from build123d import *

# Parameters (mm, degrees)
EXTRUDE_1_DEPTH = 15
EXTRUDE_START   = 8
EXTRUDE_3_DEPTH = 7
EXTRUDE_4_DEPTH = 15
EXTRUDE_5_DEPTH = 15
EXTRUDE_6_DEPTH = 15
FILLET_1_R      = 2
FILLET_2_R      = 0.8
F_2_0MM_1_D     = 2.2
F_2_0MM_1_DEPTH = 1.5
F_2_0MM_1_TIP   = 0.660946681
F_2_0MM_2_D     = 2.2
F_2_0MM_2_DEPTH = 1.5
F_2_0MM_2_TIP   = 0.660946681


with BuildPart() as part:
    # 草图1 → 凸台-拉伸1 (new body)
    with BuildSketch(Plane(origin=(0, 0, 0), x_dir=(1, 0, 0), z_dir=(0, 1, 0))):
        Polygon((49.5194763, 27.3201645), (0, 0), (14.2759212, -89.0995664), (44.3217232, -113.2519378), (135.6782768, -113.2519378), (165.7240788, -89.0995664), (180, 0), (130.4805237, 27.3201645), (90, 17.2995935), align=None)
        Polygon((6.502592683, -14.920940874), (11.7659704, -11.9027565), (24.4692995, -92.1170773), (17.9120995, -86.965507524), align=None, mode=Mode.SUBTRACT)
        Polygon((51.5112815, 10), (90, 0), (128.4887185, 10), (152.140164487, -3.156709279), (153.941562556, -4.158782079), (157.3669305, -6.0642288), (164.466088374, -10.013313195), (163.0222846, -19.1574054), (162.41503493, -23.003320662), (162.112651759, -24.918414423), (150.9253582, -95.7712863), (134.2722611, -109.1590702), (45.7277389, -109.1590702), (29.0746418, -95.7712863), (17.887348241, -24.918414423), (17.58496507, -23.003320662), (16.9777154, -19.1574054), (15.533911626, -10.013313195), (22.6330695, -6.0642288), (26.058437444, -4.158782079), (27.859835513, -3.156709279), align=None, mode=Mode.SUBTRACT)
        Polygon((162.0879005, -86.965507524), (155.5307005, -92.1170773), (168.2340296, -11.9027565), (173.497407317, -14.920940874), align=None, mode=Mode.SUBTRACT)
        Polygon((50.326908, 23.3565545), (90, 13.1373278), (129.673092, 23.3565545), (166.5422291, 2.924677806), (165.312614852, -5.602660324), (128.635248263, 14.72294235), (90, 4.7710495), (51.364751737, 14.72294235), (14.687385148, -5.602660324), (13.4577709, 2.924677806), align=None, mode=Mode.SUBTRACT)
    extrude(amount=EXTRUDE_1_DEPTH)

    # 草图1<4> → 凸台-拉伸3 (add)
    with BuildSketch(Plane(origin=(0, 0, 0), x_dir=(1, 0, 0), z_dir=(0, 1, 0)).offset(EXTRUDE_START)):
        Polygon((164.466088374, -10.013313195), (163.0222846, -19.1574054), (155.8678549, -15.177574667), (157.3669305, -6.0642288), align=None)
        Polygon((153.941562556, -4.158782079), (152.140164487, -3.156709279), (149.6966334, -18.0116932), (162.112651759, -24.918414423), (162.41503493, -23.003320662), (151.8119905, -17.1051116), align=None)
        Polygon((22.6330695, -6.0642288), (15.533911626, -10.013313195), (16.9777154, -19.1574054), (24.1321451, -15.177574667), align=None)
        Polygon((30.3033666, -18.0116932), (27.859835513, -3.156709279), (26.058437444, -4.158782079), (28.1880095, -17.1051116), (17.58496507, -23.003320662), (17.887348241, -24.918414423), align=None)
    extrude(amount=EXTRUDE_3_DEPTH)

    # 草图3 → 凸台-拉伸4 (add)
    with BuildSketch(Plane(origin=(0, 0, 0), x_dir=(1, 0, 0), z_dir=(0, 1, 0))):
        Polygon((115.878940082, 32.456095876), (121.872227157, 33.965105872), (122.289100924, 40.131370332), (125.576282273, 34.897725339), (131.569569347, 36.406735336), (127.607872073, 31.663154849), (130.895053422, 26.429509857), (125.159408505, 28.73146088), (121.197711231, 23.987880393), (121.614584999, 30.154144853), align=None)
    extrude(amount=EXTRUDE_4_DEPTH)

    # 草图4 → 凸台-拉伸5 (add)
    with BuildSketch(Plane(origin=(0, 0, 0), x_dir=(1, 0, 0), z_dir=(0, 1, 0))):
        Polygon((168.625201424, 5.109151957), (158.192316311, 27.022904619), (179.513278304, 15.426602313), (155.448122239, 12.276060926), (173.065400703, 28.970046279), align=None)
        Polygon((173.065400703, 28.970046279), (166.336199119, 22.593511282), (171.369395495, 19.85599565), align=None)
        Polygon((179.513278304, 15.426602313), (171.369395495, 19.85599565), (170.321206632, 14.223202586), align=None)
        Polygon((170.321206632, 14.223202586), (164.640193911, 13.479460653), (168.625201424, 5.109151957), align=None)
        Polygon((164.640193911, 13.479460653), (162.177323823, 18.652595923), (155.448122239, 12.276060926), align=None)
        Polygon((166.336199119, 22.593511282), (158.192316311, 27.022904619), (162.177323823, 18.652595923), align=None)
    extrude(amount=EXTRUDE_5_DEPTH)

    # 草图5 → 凸台-拉伸6 (add)
    with BuildSketch(Plane(origin=(0, 0, 0), x_dir=(1, 0, 0), z_dir=(0, 1, 0))):
        Polygon((145.437967888, 18.068925838), (136.74389696, 36.330386388), (154.511365288, 26.666801134), (134.457068567, 24.041349978), (149.138133954, 37.953004439), align=None)
        Polygon((143.530465967, 32.639225275), (136.74389696, 36.330386388), (140.064736554, 29.355129142), align=None)
        Polygon((149.138133954, 37.953004439), (143.530465967, 32.639225275), (147.724796281, 30.357962248), align=None)
        Polygon((154.511365288, 26.666801134), (147.724796281, 30.357962248), (146.851305561, 25.663968028), align=None)
        Polygon((146.851305561, 25.663968028), (142.117128294, 25.044183084), (145.437967888, 18.068925838), align=None)
        Polygon((142.117128294, 25.044183084), (140.064736554, 29.355129142), (134.457068567, 24.041349978), align=None)
    extrude(amount=EXTRUDE_6_DEPTH)

    # 圆角1
    # the kernel refuses this fillet: 2 mm, written as the material it adds along each edge
    with BuildSketch(Plane(origin=(121.268833448, 15, -25.039897652), x_dir=(-0.9707016379334082, 0, 0.2402880149183444), z_dir=(0, -1, 0))) as fillet_1_piece_1:
        with BuildLine():
            CenterArc((FILLET_1_R * 0.72959801192, FILLET_1_R), FILLET_1_R, 197.771167986, 72.228832014)
            Line((-FILLET_1_R * 0.222685090293, FILLET_1_R * 0.69478385816), (-FILLET_1_R * 0.241730752337, FILLET_1_R * 0.688679535323))
            Line((-FILLET_1_R * 0.241730752337, FILLET_1_R * 0.688679535323), (-FILLET_1_R * 0.0145919602384, -FILLET_1_R * 0.02))
            Line((-FILLET_1_R * 0.0145919602384, -FILLET_1_R * 0.02), (FILLET_1_R * 0.72959801192, -FILLET_1_R * 0.02))
            Line((FILLET_1_R * 0.72959801192, -FILLET_1_R * 0.02), (FILLET_1_R * 0.72959801192, 0))
        make_face()
    extrude(amount=15)
    with BuildSketch(Plane(origin=(130.355139653, 0, -27.289126864), x_dir=(-0.5318771148973955, 0, -0.8468215482900885), z_dir=(0, 1, 0))) as fillet_1_piece_2:
        with BuildLine():
            CenterArc((0.649299153, -2), FILLET_1_R, 90, 20.172783533)
            Line((-0.040405567, -0.122686121), (-0.054199661, -0.085139844))
            ThreePointArc((-0.054199661, -0.085139844), (-0.058195374, -0.048830544), (-0.03799259, 0.012512517))
            Line((-0.03799259, 0.012512517), (0, 0.04))
            Line((0, 0.04), (0.649299153, 0.04))
            Line((0.649299153, 0.04), (0.649299153, 0))
        make_face()
    extrude(amount=15)
    with BuildSketch(Plane(origin=(168.822041947, 0, -6.166940275), x_dir=(0.18294627145075168, 0, -0.9831229128457274), z_dir=(0, 1, 0))) as fillet_1_piece_3:
        with BuildLine():
            CenterArc((FILLET_1_R * 0.721961366951, -FILLET_1_R), FILLET_1_R, 90, 71.655658553)
            Line((-FILLET_1_R * 0.227220826301, -FILLET_1_R * 0.685272873726), (-FILLET_1_R * 0.246204470166, -FILLET_1_R * 0.678978331201))
            Line((-FILLET_1_R * 0.246204470166, -FILLET_1_R * 0.678978331201), (-FILLET_1_R * 0.014439227339, FILLET_1_R * 0.02))
            Line((-FILLET_1_R * 0.014439227339, FILLET_1_R * 0.02), (FILLET_1_R * 0.721961366951, FILLET_1_R * 0.02))
            Line((FILLET_1_R * 0.721961366951, FILLET_1_R * 0.02), (FILLET_1_R * 0.721961366951, 0))
        make_face()
    extrude(amount=15)
    with BuildSketch(Plane(origin=(156.29474807, 0, -13.078316465), x_dir=(-0.8755846083755204, 0, -0.4830647923166069), z_dir=(0, 1, 0)), Plane(origin=(135.180696403, 0, -24.727053647), x_dir=(-0.8755846083755225, 0, -0.4830647923166032), z_dir=(0, 1, 0))) as fillet_1_piece_4:
        with BuildLine():
            CenterArc((FILLET_1_R * 0.731143736262, -FILLET_1_R), FILLET_1_R, 90, 72.344341447)
            Line((-FILLET_1_R * 0.221752752158, -FILLET_1_R * 0.696704298814), (-FILLET_1_R * 0.240810681926, -FILLET_1_R * 0.69063838479))
            Line((-FILLET_1_R * 0.240810681926, -FILLET_1_R * 0.69063838479), (-FILLET_1_R * 0.0146228747252, FILLET_1_R * 0.02))
            Line((-FILLET_1_R * 0.0146228747252, FILLET_1_R * 0.02), (FILLET_1_R * 0.731143736262, FILLET_1_R * 0.02))
            Line((FILLET_1_R * 0.731143736262, FILLET_1_R * 0.02), (FILLET_1_R * 0.731143736262, 0))
        make_face()
    extrude(amount=15)
    with BuildSketch(Plane(origin=(145.606582968, 0, -18.975035304), x_dir=(0.8755846083755114, 0, 0.4830647923166232), z_dir=(0, 1, 0))) as fillet_1_piece_5:
        with BuildLine():
            CenterArc((FILLET_1_R * 0.721961366951, FILLET_1_R), FILLET_1_R, 198.344341447, 71.655658553)
            Line((-FILLET_1_R * 0.227220826301, FILLET_1_R * 0.685272873726), (-FILLET_1_R * 0.246204470166, FILLET_1_R * 0.678978331201))
            Line((-FILLET_1_R * 0.246204470166, FILLET_1_R * 0.678978331201), (-FILLET_1_R * 0.014439227339, -FILLET_1_R * 0.02))
            Line((-FILLET_1_R * 0.014439227339, -FILLET_1_R * 0.02), (FILLET_1_R * 0.721961366951, -FILLET_1_R * 0.02))
            Line((FILLET_1_R * 0.721961366951, -FILLET_1_R * 0.02), (FILLET_1_R * 0.721961366951, 0))
        make_face()
    extrude(amount=15)

    # 圆角2
    fillet_2_edges = [part.edges().sort_by_distance(p)[0] for p in [
        (122.286771787, 7.5, -25.291878665),
        (129.364316192, 7.5, -27.043857882),
        (167.872084093, 7.5, -6.691037191),
        (157.30763239, 7.5, -12.519502675),
        (144.792841891, 7.5, -19.423980684),
        (136.046428654, 7.5, -24.249424454),
    ]]
    fillet(fillet_2_edges, radius=FILLET_2_R)

    # Ø2.0mm 暗销孔1
    with Locations(Plane(origin=(0, 0, 0), x_dir=(0.1582065041586212, 0, 0.9874060471973565), z_dir=(-0.9874060471973565, 0, 0.1582065041586212))):
        with Locations((82.844584748, 4.5), (52.844584748, 4.5), (67.844584748, 4.5)):
            Hole(F_2_0MM_1_D / 2, depth=F_2_0MM_1_DEPTH)
            with Locations((0, 0, -(F_2_0MM_1_DEPTH + F_2_0MM_1_TIP / 2))):  # 118° drill point
                Cone(0, F_2_0MM_1_D / 2, F_2_0MM_1_TIP, mode=Mode.SUBTRACT)

    # Ø2.0mm 暗销孔2
    with Locations(Plane(origin=(175.494726368, 0, 28.118530604), x_dir=(0.15820650415862106, 0, -0.9874060471973566), z_dir=(0.9874060471973566, 0, 0.15820650415862106))):
        with Locations((-54.462210035, 4.481040738), (-39.322424853, 4.512160057), (-24.310921517, 4.409353726)):
            Hole(F_2_0MM_2_D / 2, depth=F_2_0MM_2_DEPTH)
            with Locations((0, 0, -(F_2_0MM_2_DEPTH + F_2_0MM_2_TIP / 2))):  # 118° drill point
                Cone(0, F_2_0MM_2_D / 2, F_2_0MM_2_TIP, mode=Mode.SUBTRACT)


solid = part.part
Read the model definition and answer for the solid it produces. Units are mm, in the model's axes. A direction names the side the tool comes from. Round coordinates to 2 decimals unless told otherwise and drop trailing zeros. Write each loop counter-clockwise with the first axis right and the second up, starting at its lowest first coordinate (ties: lowest second). Pieces come first, ordered by that corner, then holes. Notation, with made-up numbers: (65, 79) - (108, 79) arc R8 cw to (108, 94) - close; hole circle Ø6 at (9.25, -6.5). An arc over 180 degrees is marked (long way). Use a Markdown table: item, result.
(1) The part is cut by section C-C (y = 11). State how many separate pieces and enclosed holes the cut face has, then the cut area to 3 significant figures.
Reported:
| item | result |
|---|---|
| separate pieces | 1 |
| enclosed holes | 9 |
| area | 4,400 mm2 |
(2) Which of the six approach directions +Z, -Z, +X, -X, +Y, -Y give full straight-line access (tool end or side, diameter ignored) to faces 4 (the flat face through (18.03, 7.4, 51.45)), 5 (the flat face through (7.04, 7.4, 43.93)), 6 (the flat face through (28.2, 8, 15.6)), 7 (the flat face through (118.787, 7.395, -31.289))?
Reported:
| item | result |
|---|---|
| face 4 | +Y, -Y |
| face 5 | +Z, -X, +Y, -Y |
| face 6 | -Y |
| face 7 | -X, +Y, -Y |
(3) The part is cut by section B-B (z = 70.5). Write down the section's boundary in (x, y), then the cut area to 3 significant figures.
Reported:
| item | result |
|---|---|
| outline | (11.3, 0) - (15.3, 0) - (15.3, 15) - (11.3, 15) - close; (21.05, 0) - (25.08, 0) - (25.08, 15) - (21.05, 15) - close; (154.92, 0) - (158.95, 0) - (158.95, 15) - (154.92, 15) - close; (164.7, 0) - (168.7, 0) - (168.7, 15) - (164.7, 15) - close |
| area | 241 mm2 |
(4) The mould has two halves that part along X. Classify faces 1 (the flat face through (91, 7, 109.159)), 2 (the flat face through (108.97, 7.4, -4.93)), 3 (the flat face through (25.106, 7.395, -13.851)): released by +X, released by -X, zero draft, split by the parting line, or undercut.
Reported:
| item | result |
|---|---|
| face 1 | undercut |
| face 2 | undercut |
| face 3 | released by -X |
(5) The part is cut by section A-A (x = 66.5). Write down the section's boundary in (y, z), then the cut area to 3 significant figures.
Reported:
| item | result |
|---|---|
| outline | (0, -23.12) - (15, -23.12) - (15, -19.19) - (0, -19.19) - close; (0, -10.82) - (15, -10.82) - (15, -6.11) - (0, -6.11) - close; (0, 109.16) - (15, 109.16) - (15, 113.25) - (0, 113.25) - close |
| area | 191 mm2 |
(6) Straight lines are drawn through the part: line 1 along Z through (x, y) = (100, 10.25) (3 decimals); line 2 along X through (y, z) = (11.25, 80.5); line 3 along X through (y, z) = (2.25, 60). For each, find the intervals that lie inside material, in ascending order. Write a range as [from, to].
Reported:
| item | result |
|---|---|
| line 1 | [-19.775, -15.713], [-7.347, -2.598], [109.159, 113.252] |
| line 2 | [12.9, 16.89], [22.63, 26.66], [153.34, 157.37], [163.11, 167.1] |
| line 3 | [9.61, 13.64], [19.38, 23.43], [156.57, 160.62], [166.36, 170.39] |
(7) The part is cut by section D-D (x = 34.5). Write down the section's boundary in (y, z).
Reported:
| item | result |
|---|---|
| outline | (0, -19.03) - (15, -19.03) - (15, -14.59) - (0, -14.59) - close; (0, -5.38) - (15, -5.38) - (15, -0.54) - (0, -0.54) - close; (0, 100.13) - (15, 100.13) - (15, 105.36) - (0, 105.36) - close |
(8) Each of these flat-tipped pins is pushed along its axis until it touches: pin 1 Ø2.5 at (x, z) = (18.5, 15) entering from -Y; pin 2 Ø3 at (y, z) = (2.5, -2) entering from -X. Where does it stop, or does it pass through?
Reported:
| item | result |
|---|---|
| pin 1 | y = 8 |
| pin 2 | x = 0.91 |
